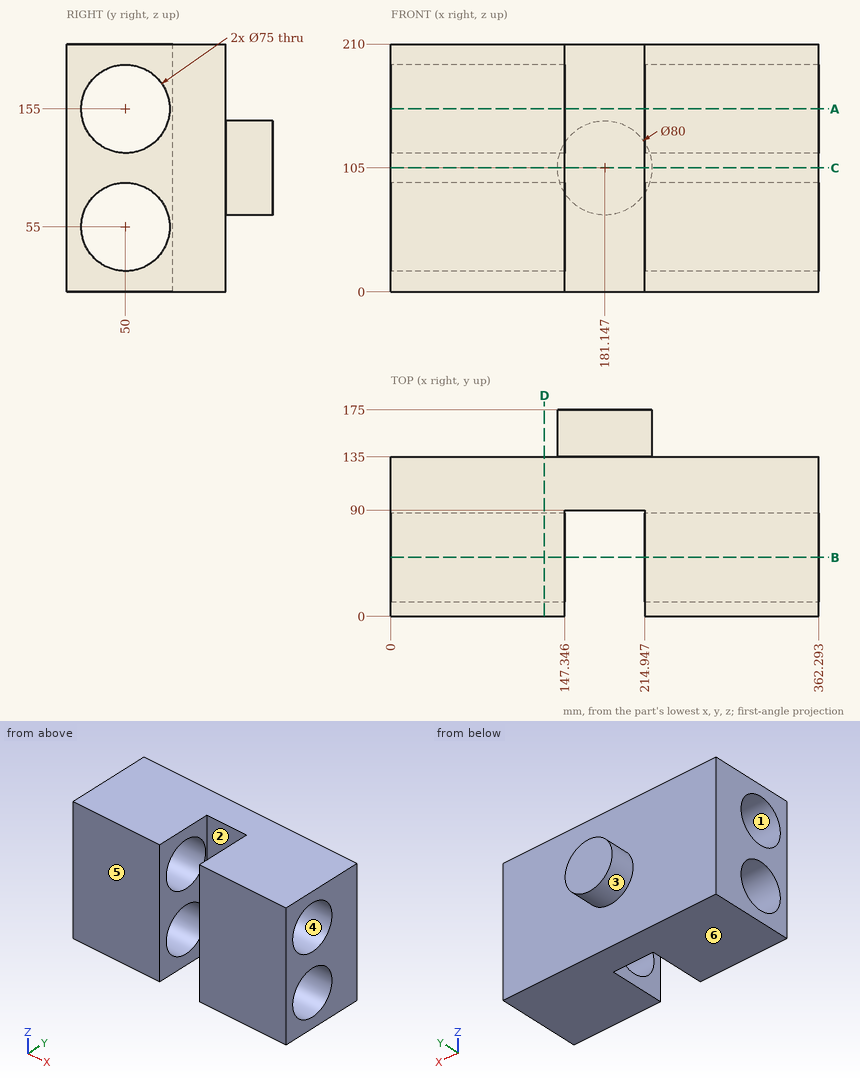
Check sheet for the drawn part. Datum: minimum x, y, z corner. Units: mm. A direction names the side the tool comes from. Coordinates: 2 decimals unless noted, no trailing zeros. Order: outer loops, then holes, each group sorted by start corner. A loop starts at its lowest first (then second) coordinate and runs counter-clockwise, first axis right, second up. Notation, with made-up numbers: (44.25, 48) -> (80.25, 48) arc R8 cw to (80.25, 59) -> close; hole circle Ø5 at (56.5, 84.5). An arc over 180 degrees is marked (long way). Use a Markdown table: item, result. Add a question column.
1. Go/stop test with flat-tipped pins: pin 1 Ø8 at (x, z) = (154.5, 144) entering from +Y; pin 2 Ø10 at (x, y) = (187.5, 100) entering from -Z; pin 3 Ø20.5 at (x, z) = (189.5, 89) entering from -Y. Record where each tip stops, or that it passes through.
2. Mould release check, pull along Z, two halves, no side actions. Record for the marked faces 4, 5 and 6: pulls with the +Z half, pulls with the -Z half, needs draft (parallel to the pull), parting line crosses it, or undercut.
3. Material ranges on L1, parallel to Z at x = 317.5, y = 50; L2, parallel to X at y = 85, z = 169; L3, parallel to Z at x = 252, y = 19, recorded low to high.
4. Cross-section at D-D (x = 130). Enter the section's corners in (y, z).
5. Cross-section at A-A (z = 155). Enter the section's corners in (x, y), and give its area (3 significant figures).
6. Cross-section at C-C (z = 105). Enter the section's corners in (x, y), and give its area (3 significant figures).
7. Cross-section at B-B (y = 50). Enter the section's corners in (x, z), and give its area (3 significant figures).
8. Set-up check for the marked faces 1, 2 and 3: record each of +Z, -Z, +X, -X, +Y, -Y from which the full face is reachable in a straight line by a thin tool's end or side.
Filled sheet:
| question | item | result |
|---|---|---|
| 1 | pin 1 | y = 135 |
| 1 | pin 2 | z = 0 |
| 1 | pin 3 | y = 90 |
| 2 | face 4 | undercut |
| 2 | face 5 | needs draft |
| 2 | face 6 | pulls with the -Z half |
| 3 | L1 | 0 to 17.5, 92.5 to 117.5, 192.5 to 210 |
| 3 | L2 | 0 to 147.35, 214.95 to 362.29 |
| 3 | L3 | 0 to 33.9, 76.1 to 133.9, 176.1 to 210 |
| 4 | outline | (0, 0) -> (135, 0) -> (135, 210) -> (0, 210) -> close; hole circle Ø75 at (50, 55); hole circle Ø75 at (50, 155) |
| 5 | outline | (0, 0) -> (147.35, 0) -> (147.35, 12.5) -> (0, 12.5) -> close; (0, 87.5) -> (147.35, 87.5) -> (147.35, 90) -> (214.95, 90) -> (214.95, 87.5) -> (362.29, 87.5) -> (362.29, 135) -> (0, 135) -> close; (214.95, 0) -> (362.29, 0) -> (362.29, 12.5) -> (214.95, 12.5) -> close |
| 5 | area | 20,700 mm2 |
| 6 | outline | (0, 0) -> (147.35, 0) -> (147.35, 90) -> (214.95, 90) -> (214.95, 0) -> (362.29, 0) -> (362.29, 135) -> (221.15, 135) -> (221.15, 175) -> (141.15, 175) -> (141.15, 135) -> (0, 135) -> close |
| 6 | area | 46,000 mm2 |
| 7 | outline | (0, 0) -> (147.35, 0) -> (147.35, 17.5) -> (0, 17.5) -> close; (0, 92.5) -> (147.35, 92.5) -> (147.35, 117.5) -> (0, 117.5) -> close; (0, 192.5) -> (147.35, 192.5) -> (147.35, 210) -> (0, 210) -> close; (214.95, 0) -> (362.29, 0) -> (362.29, 17.5) -> (214.95, 17.5) -> close; (214.95, 92.5) -> (362.29, 92.5) -> (362.29, 117.5) -> (214.95, 117.5) -> close; (214.95, 192.5) -> (362.29, 192.5) -> (362.29, 210) -> (214.95, 210) -> close |
| 7 | area | 17,700 mm2 |
| 8 | face 1 | +X, -X |
| 8 | face 2 | +Z, -Z, -Y |
| 8 | face 3 | +Y |
